Source: three-view drawing plus pictorial views. Frame: mm from the lowest corner of the part. A direction names the side the tool comes from. Give positions to 0.01 mm unless a question says otherwise; leave off trailing zeros. Loops run counter-clockwise (first coordinate to the right, second up) from the corner with the lowest first, then second, coordinate; pieces in that order, holes last.
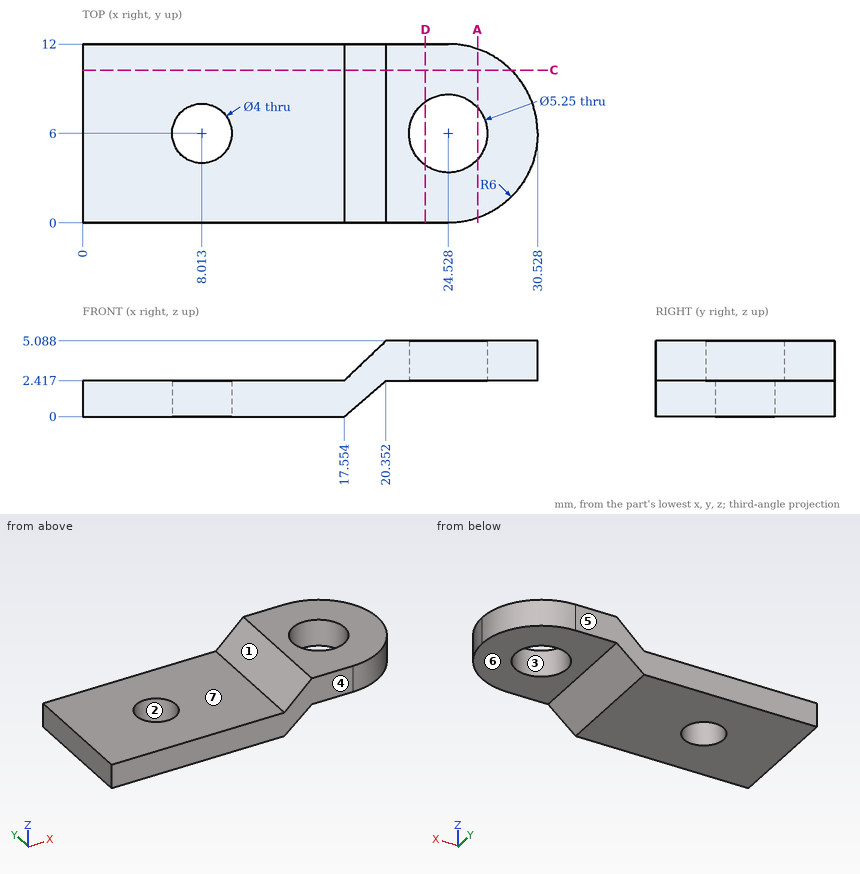
(1) Ray query, probe 1 along Z at (x, y) = (25, 9.5); probe 2 along Z at (x, y) = (12, 2); probe 3 along X at (y, z) = (4.75, 3) (1 decimal). Return the intervals inside material, ascending.
Values follow:
probe 1: z = 2.42 to 5.09
probe 2: z = 0 to 2.42
probe 3: x = 18.2 to 22.2, 26.8 to 30.4
(2) Mould query, pull axis X, two halves, no side actions, for the marked faces 1, 2, 3 and 4. Classes: +X half, -X half, draft (parallel to the pull), parting line (faces both ways), or undercut.
Values follow:
face 1: -X half
face 2: undercut
face 3: undercut
face 4: draft
(3) Cut plane D-D (x = 23). Return the cut outline in (y, z) (1 decimal).
Values follow:
outline: (0, 2.4) - (3.9, 2.4) - (3.9, 5.1) - (0, 5.1) - close; (8.1, 2.4) - (12, 2.4) - (12, 5.1) - (8.1, 5.1) - close
(4) Pin query (flat end, axial travel): pin 1 Ø3.5 at (x, y) = (11, 7) entering from +Z; pin 2 Ø2 at (x, y) = (18, 2.5) entering from +Z. Return the tip coordinate at first contact, or that it passes through.
Values follow:
pin 1: stops at z = 2.42
pin 2: stops at z = 3.8
(5) Reachability of the marked faces 5, 6 and 7 from +Z, -Z, +X, -X, +Y, -Y: full face, straight path, thin tool, end or side. Return the list, or none.
Values follow:
face 5: +Z, -Z, +X, -X, +Y
face 6: -Z, +X, +Y, -Y
face 7: +Z, -X, +Y, -Y
(6) Cut plane C-C (y = 10.25). Return the cut outline in (x, z).
Values follow:
outline: (0, 0) - (17.55, 0) - (20.35, 2.42) - (28.76, 2.42) - (28.76, 5.09) - (20.35, 5.09) - (17.55, 2.42) - (0, 2.42) - close
(7) Cut plane A-A (x = 26.5). Return the cut outline in (y, z), and give its area (3 significant figures).
Values follow:
outline: (0.33, 2.42) - (4.27, 2.42) - (4.27, 5.09) - (0.33, 5.09) - close; (7.73, 2.42) - (11.67, 2.42) - (11.67, 5.09) - (7.73, 5.09) - close
area: 21.0 mm2
